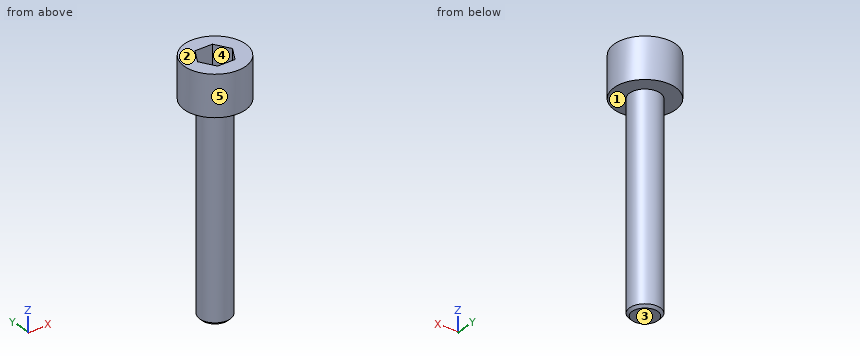
Autodesk Inventor part; units mm, degrees
ref_plane "YZ Plane" through (0, 0, 0) normal (1, 0, 0) x (0, 1, 0)
ref_plane "XZ Plane" through (0, 0, 0) normal (0, 1, 0) x (-1, 0, 0)
ref_plane "XY Plane" through (0, 0, 0) normal (0, 0, 1) x (1, 0, 0)
sketch "草图1" plane through (0, 0, 0) normal (0, 0, 1) x (1, 0, 0)
  circle A0 centre (0, 0) radius 3
  dimension "d0" = 6
extrude "拉伸1" add sketch "草图1" along normal blind 4
sketch "草图2" plane through (0, 0, 4) normal (0, 0, 1) x (1, 0, 0)
  line L0 (0.866, -1.5) -> (-0.866, -1.5)
  line L1 (-0.866, -1.5) -> (-1.7321, 0)
  line L2 (-1.7321, 0) -> (-0.866, 1.5)
  line L3 (-0.866, 1.5) -> (0.866, 1.5)
  line L4 (0.866, 1.5) -> (1.7321, 0)
  line L5 (1.7321, 0) -> (0.866, -1.5)
  line L6 (0, 0) -> (0, 1.5)
  dimension "d3" = 3
extrude "拉伸2" cut sketch "草图2" against normal blind 2.5
sketch "草图3" plane through (0, 0, 0) normal (0, 0, -1) x (-1, 0, 0)
  circle A0 centre (0, 0) radius 1.5
  dimension "d6" = 3
extrude "拉伸3" add sketch "草图3" along normal blind 20
thread "螺纹1"
chamfer "倒角1" distance 0.25 angle 45 1 edges at (1.5, 0, -20)
properties part number "刀轴拨叉紧固螺丝"
Work out the finished part from the listing and answer in its coordinate system (mm). Face numbers are marked on the shaded views. A direction names the side the tool comes from. Give positions to 0.01 mm unless a question says otherwise; leave off trailing zeros. Loops run counter-clockwise (first coordinate to the right, second up) from the corner with the lowest first, then second, coordinate; pieces in that order, holes last. Notation, with made-up numbers: (56.5, 37) - (84.5, 37) arc R18 ccw to (84.5, 68) - close; hole circle Ø7 at (5, 62.25). An arc over 180 degrees is marked (long way). Use CSV: the item, a comma, the result in double quotes. Start each with the question number.
(1) Each of these flat-tipped pins is pushed along its axis until it touches: pin 1 (1.5 mm diameter, centred on x = -2.5, y = 2, fed in from -Z); pin 2 (2 mm diameter, centred on y = 1, z = -14.5, fed in from -X); pin 3 (0.5 mm diameter, centred on x = -0.5, z = 3, fed in from -Y). Where does it stop, or does it pass through?
(2) Find the intervals of material crossed by L1, parallel to Z at x = 2, y = 0.45; L2, parallel to Y at x = 0.45, z = 2.5; L3, parallel to Z at x = 0.4, y = -0.7, in increasing order.
(3) Find section C-C, the plane z = -14.75. Determine the outline of the cut face in (x, y), plus the area to 3 significant figures.
(4) A tool of negligible diameter and unlimited length cuts with its end or side. For the marked faces 1 and 2, from which of +Z, -Z, +X, -X, +Y, -Y can it reach the whole face along a straight path? Write none if from no direction.
(5) Find section D-D, the plane y = -2.3. Determine the outline of the cut face in (x, z).
(6) Find section B-B, the plane z = 2.25. Determine the outline of the cut face in (x, y).
(7) Determine the mould class of the marked faces 3, 4 and 5 for opening direction X: released by +X, released by -X, zero draft, split by the parting line, or undercut.
(8) Find section A-A, the plane x = 0. Determine the outline of the cut face in (y, z), plus the area to 3 significant figures.
Results found:
1,pin 1,"z = 0"
1,pin 2,"x = -1.5"
1,pin 3,"y = -2.99"
2,L1,"0 to 4"
2,L2,"-2.97 to -1.5, 1.5 to 2.97"
2,L3,"-20 to 1.5"
3,outline,"circle Ø3 at (0, 0)"
3,area,"7.07 mm^2"
4,face 1,"-Z"
4,face 2,"+Z, +X, -X, +Y, -Y"
5,outline,"(-1.93, 0) - (1.93, 0) - (1.93, 4) - (-1.93, 4) - close"
6,outline,"circle Ø6 at (0, 0); hole (-1.73, 0) - (-0.87, -1.5) - (0.87, -1.5) - (1.73, 0) - (0.87, 1.5) - (-0.87, 1.5) - close"
7,face 3,"zero draft"
7,face 4,"undercut"
7,face 5,"split by the parting line"
8,outline,"(-3, 0) - (-1.5, 0) - (-1.5, -19.75) - (-1.25, -20) - (1.25, -20) - (1.5, -19.75) - (1.5, 0) - (3, 0) - (3, 4) - (1.5, 4) - (1.5, 1.5) - (-1.5, 1.5) - (-1.5, 4) - (-3, 4) - close"
8,area,"76.4 mm^2"
